Part model, mm, in its own coordinate system. A direction names the side the tool comes from. Coordinates: 2 decimals unless noted, no trailing zeros. Write each loop counter-clockwise with the first axis right and the second up, starting at its lowest first coordinate (ties: lowest second). Pieces come first, ordered by that corner, then holes. Notation, with made-up numbers: (73, 16) - (78, 16) arc R8 cw to (78, 23) - close; hole circle Ø10 at (42.5, 40). An arc over 180 degrees is marked (long way). Write each question's results on one line, items separated by ' | '.
from build123d import *

# Parameters (mm, degrees)
PAD_DEPTH            = 9.020639
POCKET_DEPTH         = 2.7
SKETCH003_R          = 1.75
POCKET001_DEPTH      = 6.051
POCKET001_DEPTH_BACK = -6.051
FILLET_R             = 5


with BuildPart() as part:
    # Sketch001 → Pad (new body, symmetric)
    with BuildSketch(Plane.XY):
        with BuildLine():
            ThreePointArc((2, 10.753118), (0, 18.324836), (-2, 10.753118))
            Line((-2, 10.753118), (-2, -11.595564))
            Line((-6.0498, -11.595564), (-2, -11.595564))
            Line((-6.0498, 14.225598), (-6.0498, -11.595564))
            ThreePointArc((6.049634, 14.208289), (0.008655, 20.32483), (-6.0498, 14.225598))
            Line((6.049634, 14.208289), (6.049634, -11.595564))
            Line((2, -11.595564), (6.049634, -11.595564))
            Line((2, 10.753118), (2, -11.595564))
        make_face()
    extrude(amount=PAD_DEPTH, both=True)

    # Sketch002 → Pocket (cut, symmetric)
    with BuildSketch(Plane.YZ):
        with BuildLine():
            ThreePointArc((0.277273, -8.220161), (8.224836, 1e-06), (0.277271, 8.220161))
            Line((-11.595564, 8.620639), (0.277271, 8.220161))
            Line((-11.595564, 8.620639), (-11.595564, -8.620639))
            Line((-11.595564, -8.620639), (0.277273, -8.220161))
        make_face()
    extrude(amount=POCKET_DEPTH, both=True, mode=Mode.SUBTRACT)

    # Sketch003 → Pocket001 (cut, two sides)
    with BuildSketch(Plane.YZ) as pocket001_sk:
        Circle(SKETCH003_R)
    extrude(amount=-POCKET001_DEPTH, mode=Mode.SUBTRACT)
    extrude(pocket001_sk.sketch, amount=-POCKET001_DEPTH_BACK, mode=Mode.SUBTRACT)

    # Fillet
    fillet_edges = [part.edges().sort_by_distance(p)[0] for p in [
        (2, 10.753118, 0),
        (-2, 10.753118, 0),
    ]]
    fillet(fillet_edges, radius=FILLET_R)


solid = part.part
(1) Saw through at A-A on y = 5.5. Write the cut outline in (x, z), then the cut area to 3 significant figures.
Return value:
outline: (-6.05, -9.02) - (-2, -9.02) - (-2, -6.12) - (-2.7, -6.12) - (-2.7, 6.12) - (-2, 6.12) - (-2, 9.02) - (-6.05, 9.02) - close; (2, -9.02) - (6.05, -9.02) - (6.05, 9.02) - (2, 9.02) - (2, 6.12) - (2.7, 6.12) - (2.7, -6.12) - (2, -6.12) - close | area: 129 mm^2
(2) 3-axis set-ups, long thin cutter, end or side, ignore diameter. For faces 1 (the cylindrical face through (-2.3, 10.24, -0.13)), 2 (the flat face through (2.7, -2, 0)), 3 (the flat face through (2, 8.2, 2)): which of +Z, -Z, +X, -X, +Y, -Y reach the whole face in a straight line?
Return value:
face 1: +Z, -Z | face 2: -Y | face 3: +Z, -Z, -Y
(3) Saw through at B-B on z = 0. Write the cut outline in (x, y), then the cut area to 3 significant figures.
Return value:
outline: (-6.05, -11.6) - (-2.7, -11.6) - (-2.7, -1.75) - (-6.05, -1.75) - close; (-6.05, 1.75) - (-2.7, 1.75) - (-2.7, 8.22) - (-2, 8.22) - (-2, 8.54) arc R5 ccw to (-3.13, 11.71) arc R4.05 cw (long way) to (3.13, 11.71) arc R5 ccw to (2, 8.54) - (2, 8.22) - (2.7, 8.22) - (2.7, 1.75) - (6.05, 1.75) - (6.05, 14.21) arc R6.05 ccw (long way) to (-6.05, 14.23) - close; (2.7, -11.6) - (6.05, -11.6) - (6.05, -1.75) - (2.7, -1.75) - close | area: 179 mm^2
(4) Two-plate mould, pull along Z, no slides. Class faces 4 (the flat face through (-3, 5, 9.021)), 5 (the cylindrical face through (-2.345, 8.223, -0.177)), 6 (the flat face through (-2, 8.2, 2)): released by +Z, released by -Z, zero draft, split by the parting line, or undercut.
Return value:
face 4: released by +Z | face 5: undercut | face 6: zero draft
(5) Saw through at D-D on z = 2.5. Write the cut outline in (x, y).
Return value:
outline: (-6.05, -11.6) - (-2.7, -11.6) - (-2.7, 7.84) - (-2, 7.84) - (-2, 8.54) arc R5 ccw to (-3.13, 11.71) arc R4.05 cw (long way) to (3.13, 11.71) arc R5 ccw to (2, 8.54) - (2, 7.84) - (2.7, 7.84) - (2.7, -11.6) - (6.05, -11.6) - (6.05, 14.21) arc R6.05 ccw (long way) to (-6.05, 14.23) - close
(6) Flat gauge pin, fed straight in: P1, Ø5, axis at x = 0, y = 14.27, coming from the -Z side. Where does the tip first touch, or does it go through?
Return value:
P1: passes through
(7) Saw through at C-C on y = 1. Write the cut outline in (x, z).
Return value:
outline: (-6.05, -9.02) - (-2, -9.02) - (-2, -8.16) - (-2.7, -8.16) - (-2.7, -1.44) - (-6.05, -1.44) - close; (-6.05, 1.44) - (-2.7, 1.44) - (-2.7, 8.16) - (-2, 8.16) - (-2, 9.02) - (-6.05, 9.02) - close; (2, -9.02) - (6.05, -9.02) - (6.05, -1.44) - (2.7, -1.44) - (2.7, -8.16) - (2, -8.16) - close; (2, 8.16) - (2.7, 8.16) - (2.7, 1.44) - (6.05, 1.44) - (6.05, 9.02) - (2, 9.02) - close
(8) Wall check: line 1 (Z direction, x = -4.85, y = 0); line 2 (X direction, y = -5, z = 4.5); line 3 (X direction, y = 7.5, z = -6.5). Give the ranges that are in metal, low to high. Write a range as from..to.
Return value:
line 1: z = -9.02..-1.75, 1.75..9.02 | line 2: x = -6.05..-2.7, 2.7..6.05 | line 3: x = -6.05..-2, 2..6.05
